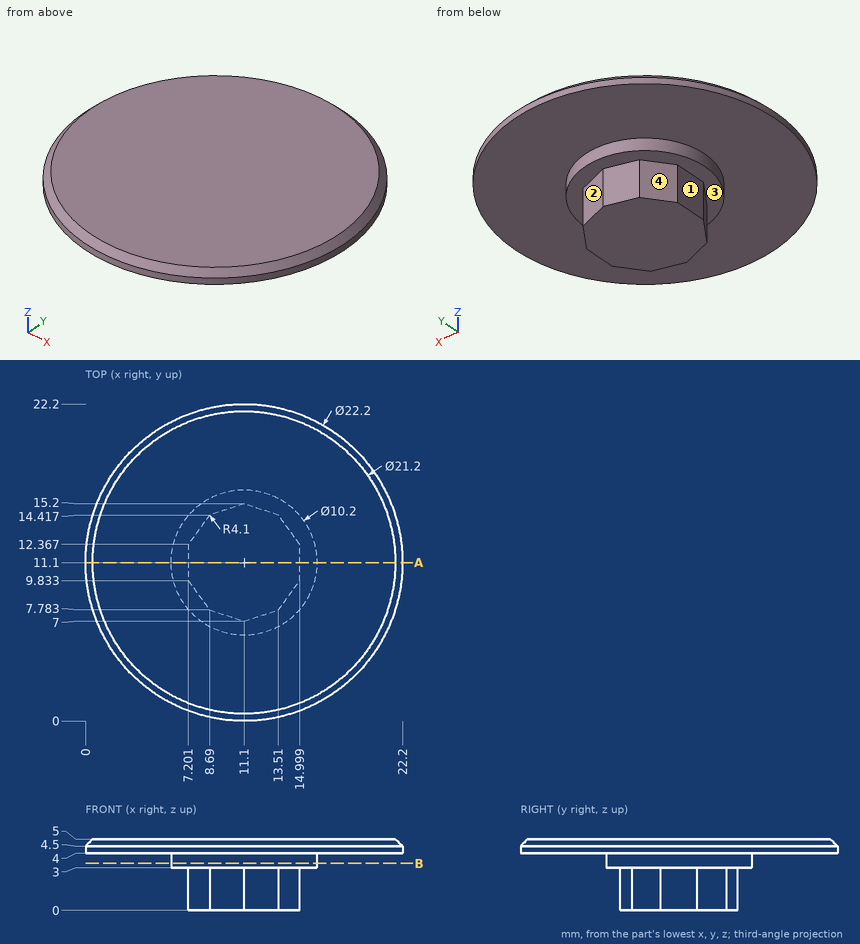
The figure shows three views and two pictorial views of one solid part (mm, origin at its lowest corner). Answer the questions. A direction names the side the tool comes from. Round coordinates to 2 decimals unless told otherwise and drop trailing zeros. Write each loop counter-clockwise with the first axis right and the second up, starting at its lowest first coordinate (ties: lowest second). Pieces come first, ordered by that corner, then holes. Notation, with made-up numbers: (13, 14.5) -> (52, 14.5) arc R14 ccw to (52, 21.5) -> close; hole circle Ø11 at (72.5, 52.5). An arc over 180 degrees is marked (long way). Write each question's results on one line, items separated by ' | '.
Q1. Straight lines are drawn through the part: line 1 along Z through (x, y) = (8, 13.75); line 2 along Z through (x, y) = (1.5, 12.25); line 3 along X through (y, z) = (11.75, 3.4). For each, find the intervals that lie inside material, in ascending order. Write a range as [from, to].
Data:
line 1: [3, 5] | line 2: [4, 5] | line 3: [6.04, 16.16]
Q2. Flat-ended cylindrical pins translate along their axes: P1, Ø1.5, axis at y = 15, z = 3.5, coming from the -X side (1 decimal); P2, Ø1, axis at x = 19, z = 2, coming from the +Y side; P3, Ø3, axis at y = 11, z = 1, coming from the +X side; P4, Ø1.5, axis at x = 3.5, z = 4.5, coming from the -Y side (1 decimal). Find the tip coordinate at first contact, or state that the pin passes through.
Data:
P1: x = 0.5 | P2: through | P3: x = 15 | P4: y = 2.4
Q3. Section B-B, the plane z = 3.3 is taken. Write down the section's boundary in (x, y), then the cut area to 3 significant figures.
Data:
outline: circle Ø10.2 at (11.1, 11.1) | area: 81.7 mm^2
Q4. Which of the six approach directions +Z, -Z, +X, -X, +Y, -Y give full straight-line access (tool end or side, diameter ignored) to the marked faces 1, 2, 3 and 4?
Data:
face 1: -Z, -X, +Y, -Y | face 2: -Z, +X, +Y | face 3: -Z | face 4: -Z, -X, +Y
Q5. Section A-A, the plane y = 11.1 is taken. Write down the section's boundary in (x, z).
Data:
outline: (0, 4) -> (6, 4) -> (6, 3) -> (7.2, 3) -> (7.2, 0) -> (15, 0) -> (15, 3) -> (16.2, 3) -> (16.2, 4) -> (22.2, 4) -> (22.2, 4.5) -> (21.7, 5) -> (0.5, 5) -> (0, 4.5) -> close
